Geometry: final body of the model. Coordinates: model frame, mm. A direction names the side the tool comes from. Coordinates: 2 decimals unless noted, no trailing zeros. Loops run counter-clockwise (first coordinate to the right, second up) from the corner with the lowest first, then second, coordinate; pieces in that order, holes last. Notation, with made-up numbers: (-32, -23) - (0, -23) arc R21 ccw to (0, 4) - close; hole circle Ø9 at (5.5, 21). An arc over 180 degrees is marked (long way). Put each result on its own line as item: value. Start each with the question number.
1) Section D-D on x = -25. Output: boundary loops of the cut face in (y, z), and give its area (3 significant figures).
2) Contact query for flat-ended pins moving along their axis: pin 1 Ø5 at (y, z) = (5.5, 7) entering from -X; pin 2 Ø2 at (x, y) = (-25.5, 12.5) entering from +Z; pin 3 Ø4.5 at (x, z) = (-8, 11.5) entering from +Y; pin 4 Ø3 at (x, y) = (34, 19) entering from -Z. Output: stop coordinate, or through.
3) Reachability of faces 1 (the flat face through (-21, 0, 9)), 2 (the flat face through (0, -19, 9)), 3 (the flat face through (21, 0, 9)), 4 (the flat face through (0, 19, 9)) from +Z, -Z, +X, -X, +Y, -Y: full face, straight path, thin tool, end or side. Return the list, or none.
4) Section A-A on x = 1. Output: boundary loops of the cut face in (y, z).
5) Section C-C on z = 10.25. Output: boundary loops of the cut face in (x, y).
6) Material intervals for line 1 along Y through (x, z) = (-34, 0.55); line 2 along Z through (x, y) = (32.5, 18); line 3 along X through (y, z) = (4.5, 5.5), sorted ascending. Write a range as from..to.
7) Section B-B on y = 7. Output: boundary loops of the cut face in (x, z).
8) Draft query along X for faces 5 (the flat face through (-1, -20, 1)), 6 (the cylindrical face through (-35.65, -18.93, 0.49)), 7 (the cylindrical face through (36.14, 21.1, 0.49)). Return one class per face: +X half, -X half, draft (parallel to the pull), parting line (faces both ways), or undercut.
```python
from build123d import *

# Parameters (mm, degrees)
CROQUIS1_R              = 1.65
SALIENTE_EXTRUIR1_DEPTH = 1
CROQUIS3_W              = 42
CROQUIS3_H              = 38
SALIENTE_EXTRUIR2_DEPTH = 16.5
REDONDEO1_R             = 1


with BuildPart() as part:
    # Croquis1 → Saliente-Extruir1 (new body)
    with BuildSketch(Plane(origin=(0, 0, 0), x_dir=(0, 1, 0), z_dir=(0, 0, 1))):
        with BuildLine():
            Line((-19, -37), (19, -37))
            ThreePointArc((19, -37), (21.121320344, -36.121320344), (22, -34))
            Line((22, -34), (22, 34))
            ThreePointArc((22, 34), (21.121320344, 36.121320344), (19, 37))
            Line((19, 37), (-19, 37))
            ThreePointArc((-19, 37), (-21.121320344, 36.121320344), (-22, 34))
            Line((-22, 34), (-22, -34))
            ThreePointArc((-22, -34), (-21.121320344, -36.121320344), (-19, -37))
        make_face()
        with Locations(Location((-19, 34, 0), (0, 0, 270))):
            Circle(CROQUIS1_R, mode=Mode.SUBTRACT)
        with Locations(Location((19, 34, 0), (0, 0, 270))):
            Circle(CROQUIS1_R, mode=Mode.SUBTRACT)
        with Locations(Location((19, -34, 0), (0, 0, 270))):
            Circle(CROQUIS1_R, mode=Mode.SUBTRACT)
        with Locations(Location((-19, -34, 0), (0, 0, 270))):
            Circle(CROQUIS1_R, mode=Mode.SUBTRACT)
    extrude(amount=SALIENTE_EXTRUIR1_DEPTH)

    # Croquis3 → Saliente-Extruir2 (add)
    with BuildSketch(Plane.XY.offset(1)):
        Rectangle(CROQUIS3_W, CROQUIS3_H)
    extrude(amount=SALIENTE_EXTRUIR2_DEPTH)

    # Redondeo1
    redondeo1_edges = [part.edges().sort_by_distance(p)[0] for p in [
        (0, 19, 17.5),
        (0, -19, 17.5),
    ]]
    fillet(redondeo1_edges, radius=REDONDEO1_R)


solid = part.part
```
Answer block:
1. outline: (-22, 0) - (22, 0) - (22, 1) - (-22, 1) - close
1. area: 44.0 mm²
2. pin 1: stops at x = -21
2. pin 2: stops at z = 1
2. pin 3: stops at y = 19
2. pin 4: passes through
3. face 1: +Z, -X, +Y, -Y
3. face 2: +Z, +X, -X, -Y
3. face 3: +Z, +X, +Y, -Y
3. face 4: +Z, +X, -X, +Y
4. outline: (-22, 0) - (22, 0) - (22, 1) - (19, 1) - (19, 16.5) arc R1 ccw to (18, 17.5) - (-18, 17.5) arc R1 ccw to (-19, 16.5) - (-19, 1) - (-22, 1) - close
5. outline: (-21, -19) - (21, -19) - (21, 19) - (-21, 19) - close
6. line 1: y = -22..-20.65, -17.35..17.35, 20.65..22
6. line 2: z = 0..1
6. line 3: x = -21..21
7. outline: (-37, 0) - (37, 0) - (37, 1) - (21, 1) - (21, 17.5) - (-21, 17.5) - (-21, 1) - (-37, 1) - close
8. face 5: draft
8. face 6: undercut
8. face 7: +X half
